```python
from build123d import *

# Parameters (mm, degrees)
F0_W      = 40
F0_H      = 44
F1_DEPTH  = 44
F2_W      = 40
F2_H      = 40
F3_DEPTH  = 36
F5_DEPTH  = 5
F7_DEPTH  = 5
F8_R      = 15
F9_R      = 5
F11_DEPTH = 5


# Not quite as in the source:
# - a feature names something its author has since deleted; it is built from what else it names


with BuildPart() as f1:
    # F0 (on Top) → F1 (new body)
    with BuildSketch(Plane.XY):
        with Locations((20, 22)):
            Rectangle(F0_W, F0_H)
    extrude(amount=F1_DEPTH)

    # F2 (on face) → F3 (cut)
    with BuildSketch(Plane.YZ.offset(40)):
        with Locations((24, 20)):
            Rectangle(F2_W, F2_H)
    extrude(amount=-F3_DEPTH, mode=Mode.SUBTRACT)

    # F4 (on face) → F5 (cut)
    with BuildSketch(Plane.YZ.offset(40)):
        Polygon((2, 42), (2, 0), (4, 0), (4, 40), (22.5, 40), (22.5, 42), align=None)
    extrude(amount=-F5_DEPTH, mode=Mode.SUBTRACT)

    # F6 (on face) → F7 (cut)
    with BuildSketch(Plane(origin=(0, 44, 0), x_dir=(-1, 0, 0), z_dir=(0, 1, 0))):
        Polygon((-4, 40), (-4, 0), (-2, 0), (-2, 42), (-22.5, 42), (-22.5, 40), align=None)
    extrude(amount=-F7_DEPTH, mode=Mode.SUBTRACT)

    # F8
    f8_edges = [f1.edges().sort_by_distance(p)[0] for p in [
        (40, 44, 42),
    ]]
    fillet(f8_edges, radius=F8_R)

    # F9
    f9_edges = [f1.edges().sort_by_distance(p)[0] for p in [
        (0, 22, 44),
        (20, 0, 44),
        (0, 0, 22),
    ]]
    fillet(f9_edges, radius=F9_R)

    # F10 (on face) → F11 (cut)
    with BuildSketch(Plane(origin=(0, 0, 0), x_dir=(1, 0, 0), z_dir=(0, 0, -1))):
        Polygon((35, -4), (35, -2), (2, -2), (2, -39), (4, -39), (4, -4), align=None)
    extrude(amount=-F11_DEPTH, mode=Mode.SUBTRACT)


solid = f1.part
```
Work out the finished part from the listing and answer in its coordinate system (mm). A direction names the side the tool comes from. Round coordinates to 2 decimals unless told otherwise and drop trailing zeros. Write each loop counter-clockwise with the first axis right and the second up, starting at its lowest first coordinate (ties: lowest second). Pieces come first, ordered by that corner, then holes. Notation, with made-up numbers: (-19, -16.75) -> (20, -16.75) arc R14 cw to (20, -10.75) -> close; hole circle Ø6 at (31.5, 22). An arc over 180 degrees is marked (long way). Write each question's results on one line, items separated by ' | '.
1) Which of the six approach directions +Z, -Z, +X, -X, +Y, -Y give full straight-line access (tool end or side, diameter ignored) to faces 1 (the flat face through (38, 12, 42)), 2 (the flat face through (22, 24, 40)), 3 (the flat face through (12, 42, 42))?
Findings:
face 1: -Z, +X | face 2: -Z, +X, +Y | face 3: -Z, +Y
2) The part is cut by section C-C (z = 29.5). Write down the section's boundary in (x, y), and give its area (3 significant figures).
Findings:
outline: (0, 5) arc R5 ccw to (5, 0) -> (40, 0) -> (40, 2) -> (35, 2) -> (35, 4) -> (4, 4) -> (4, 39) -> (2, 39) -> (2, 44) -> (0, 44) -> close | area: 295 mm²
3) Consider line 1 along X through (y, z) = (22.5, 21.5); line 2 along Z through (x, y) = (14, 15.5). Determine where each line is inside the solid, lowest interval first. Write a range as [from, to].
Findings:
line 1: x = [0, 4] | line 2: z = [40, 44]
4) The part is cut by section D-D (x = 29). Write down the section's boundary in (y, z).
Findings:
outline: (0, 0) -> (2, 0) -> (2, 5) -> (4, 5) -> (4, 40) -> (43.46, 40) -> (43.46, 44) -> (5, 44) arc R5 ccw to (0, 39) -> close
5) The part is cut by section B-B (x = 33). Write down the section's boundary in (y, z).
Findings:
outline: (0, 0) -> (2, 0) -> (2, 5) -> (4, 5) -> (4, 40) -> (41.69, 40) -> (41.69, 44) -> (5, 44) arc R5 ccw to (0, 39) -> close
6) For a pull along X with two mould halves and no side action, classify faces 4 (the flat face through (1, 12, 0)), 5 (the flat face through (3, 39, 30)), 6 (the flat face through (35, 3, 29)) as +X half, -X half, draft (parallel to the pull), parting line (faces both ways), or undercut.
Findings:
face 4: draft | face 5: undercut | face 6: +X half
7) Flat-ended cylindrical pins translate along their axes: pin 1 (0.6 mm diameter, centred on y = 42, z = 41, fed in from -X); pin 2 (21 mm diameter, centred on y = 31.5, z = 21, fed in from +X); pin 3 (22.5 mm diameter, centred on x = 16.5, z = 14.5, fed in from +Y). Find the tip coordinate at first contact, or state that the pin passes through.
Findings:
pin 1: stops at x = 0.3 | pin 2: stops at x = 4 | pin 3: stops at y = 4
8) The part is cut by section A-A (y = 9). Write down the section's boundary in (x, z), and give its area (3 significant figures).
Findings:
outline: (0, 0) -> (2, 0) -> (2, 5) -> (4, 5) -> (4, 40) -> (35, 40) -> (35, 42) -> (40, 42) -> (40, 44) -> (5, 44) arc R5 ccw to (0, 39) -> close | area: 295 mm²
